Check sheet for the drawn part. Datum: minimum x, y, z corner. Units: mm. A direction names the side the tool comes from. Give positions to 0.01 mm unless a question says otherwise; leave off trailing zeros. Loops run counter-clockwise (first coordinate to the right, second up) from the corner with the lowest first, then second, coordinate; pieces in that order, holes last.
1. Cross-section at A-A, the plane z = 12.5. Record the cut outline in (x, y), plus the area to 3 significant figures.
2. Cross-section at D-D, the plane x = 22. Record the cut outline in (y, z).
3. Material ranges on L1, parallel to Z at x = 11.75, y = 12.5; L2, parallel to Z at x = 24.75, y = 12.5; L3, parallel to X at y = 15.5, z = 10.25, recorded low to high.
4. Tool access check on the marked faces 1 and 2. Record the directions out of +Z, -Z, +X, -X, +Y, -Y that give a thin tool (end or side, any length) a straight path to the whole face; none if there is none.
5. Go/stop test with flat-tipped pins: pin 1 Ø8 at (x, z) = (13.5, 20) entering from +Y; pin 2 Ø6 at (x, y) = (9.5, 13.5) entering from -Z; pin 3 Ø1 at (x, y) = (25.5, 19.5) entering from +Z; pin 4 Ø1.5 at (x, z) = (16, 4) entering from -Y. Record where each tip stops, or that it passes through.
6. Cross-section at C-C, the plane x = 7. Record the cut outline in (y, z), plus the area to 3 significant figures.
7. Release check for a two-part mould opening along Z. For the marked faces 3, 4 and 5 record: +Z half, -Z half, draft (parallel to the pull), parting line (faces both ways), or undercut.
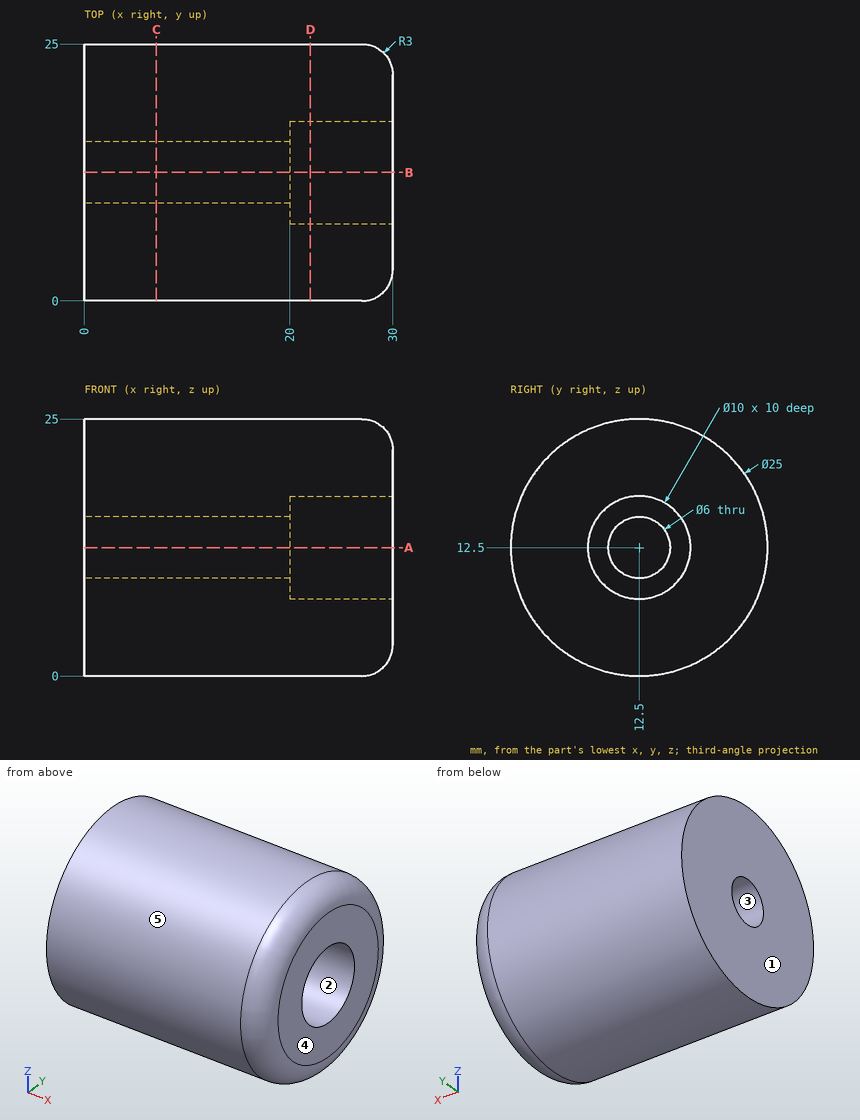
Result:
1. outline: (0, 0) - (27, 0) arc R3 ccw to (30, 3) - (30, 7.5) - (20, 7.5) - (20, 9.5) - (0, 9.5) - close; (0, 15.5) - (20, 15.5) - (20, 17.5) - (30, 17.5) - (30, 22) arc R3 ccw to (27, 25) - (0, 25) - close
1. area: 526 mm2
2. outline: circle Ø25 at (12.5, 12.5); hole circle Ø10 at (12.5, 12.5)
3. L1: z = 0 to 9.5, 15.5 to 25
3. L2: z = 0 to 7.5, 17.5 to 25
3. L3: x = 0 to 20
4. face 1: +Z, -Z, -X, +Y, -Y
4. face 2: +X
5. pin 1: stops at y = 24.5
5. pin 2: stops at z = 0
5. pin 3: stops at z = 23.18
5. pin 4: stops at y = 2.69
6. outline: circle Ø25 at (12.5, 12.5); hole circle Ø6 at (12.5, 12.5)
6. area: 463 mm2
7. face 3: undercut
7. face 4: draft
7. face 5: parting line
